Autodesk Inventor part; units mm, degrees
ref_plane "YZ Plane" through (0, 0, 0) normal (1, 0, 0) x (0, 1, 0)
ref_plane "XZ Plane" through (0, 0, 0) normal (0, 1, 0) x (-1, 0, 0)
ref_plane "XY Plane" through (0, 0, 0) normal (0, 0, 1) x (1, 0, 0)
sketch "Sketch1" plane through (0, 0, 0) normal (0, 1, 0) x (-1, 0, 0)
  line L0 (35.2615, 31.9433) -> (-167.9385, 31.9433)
  line L1 (-167.9385, 31.9433) -> (-167.9385, -69.6567)
  line L2 (-167.9385, -69.6567) -> (35.2615, -69.6567)
  line L3 (35.2615, -69.6567) -> (35.2615, 31.9433)
  line L4 (-167.9385, 31.9433) -> (-218.7385, 31.9433)
  line L5 (-218.7385, 31.9433) -> (-218.7385, 6.5433)
  line L6 (-218.7385, 6.5433) -> (-167.9385, 6.5433)
  line L7 (-167.9385, 6.5433) -> (-167.9385, 31.9433)
  line L8 (-167.9385, -69.6567) -> (-218.7385, -69.6567)
  line L9 (-218.7385, -69.6567) -> (-218.7385, -44.2567)
  line L10 (-218.7385, -44.2567) -> (-167.9385, -44.2567)
  line L11 (-167.9385, -44.2567) -> (-167.9385, -69.6567)
  point P0 (0, 0)
  point P1 (-167.9385, 6.5433)
  dimension "d0" = 101.6
  dimension "d1" = 203.2
  dimension "d2" = 50.8
  dimension "d3" = 50.8
extrude "Extrusion1" add sketch "Sketch1" along normal blind 38.1 contours L1 L6 L5 L4 | L8 L9 L10 L1
extrude "Extrusion2" add sketch "Sketch1" along normal blind 25.4 contours L3 L2 L1 L0
sketch "Sketch2" plane through (167.9385, 38.1, 31.9433) normal (0, 0, 1) x (1, 0, 0)
  line L0 (50.8, -38.1) -> (50.8, 0) construction
  line L1 (0, 0) -> (50.8, 0) construction
  line L2 (50.8, -19.05) -> (31.75, -19.05) construction
  line L3 (31.75, -19.05) -> (31.75, 0) construction
  line L4 (31.75, 0) -> (50.8, 0) construction
  line L5 (50.8, 0) -> (50.8, -19.05) construction
  circle A0 centre (31.75, -19.05) radius 12.7
  point P0 (-167.9385, -38.1)
  dimension "d8" = 25.4
extrude "Extrusion3" add sketch "Sketch2" against normal through all
fillet "Fillet1" radius 12.7 6 edges at (167.9385, 38.1, 19.2433) (167.9385, 38.1, -56.9567) (218.7385, 38.1, 19.2433) (218.7385, 38.1, -56.9567) (218.7385, 0, 19.2433) (218.7385, 0, -56.9567)
fillet "Fillet2" radius 6.35 2 edges at (-35.2615, 25.4, -18.8567) (-35.2615, 0, -18.8567)
properties part number "Pedals"
Source: CAD feature listing. Evaluate the final solid. Frame: model axes, mm. A direction names the side the tool comes from. Give positions to 0.01 mm unless a question says otherwise; leave off trailing zeros. Loops run counter-clockwise (first coordinate to the right, second up) from the corner with the lowest first, then second, coordinate; pieces in that order, holes last. Notation, with made-up numbers: (31, 74.25) -> (83, 74.25) arc R16 cw to (83, 97.25) -> close; hole circle Ø1 at (-2.75, 58.25). An arc over 180 degrees is marked (long way). Put each result on its own line as item: value. Start each with the question number.
1) Contact query for flat-ended pins moving along their axis: P1, Ø1.5, axis at y = 33, z = -48.5, coming from the +X side; P2, Ø2, axis at x = 176.5, z = 5.5, coming from the +Y side; P3, Ø10, axis at x = -0.5, z = -46, coming from the +Y side; P4, Ø2, axis at y = 33.5, z = -56, coming from the -X side. Output: stop coordinate, or through.
2) Cut plane B-B (y = 23). Return loops of the section in (x, z), then the cut area to 3 significant figures.
3) Cut plane D-D (x = 18). Return loops of the section in (y, z).
4) Reachability of faces 1 (the face through (188, 10, 6.543)), 2 (the face through (167.938, 13, -19)), 3 (the face through (71, 25.4, -18)) from +Z, -Z, +X, -X, +Y, -Y: full face, straight path, thin tool, end or side. Return the list, or none.
5) Material intervals for probe 1 along Z at (x, y) = (194, 35); probe 2 along X at (y, z) = (18, -29); probe 3 along Y at (x, z) = (103, -43.5), sorted ascending.
6) Draft query along Z for faces 4 (the face through (90, 15, 31.943)), 5 (the face through (90, 0, -18)), 6 (the face through (188, 10, -44.257)). Return one class per face: released by +Z, released by -Z, zero draft, split by the parting line, or undercut.
7) Cut plane A-A (z = -13). Return loops of the section in (x, y), then the cut area to 3 significant figures.
Results are:
1. P1: stops at x = 216.73
1. P2: passes through
1. P3: stops at y = 25.4
1. P4: stops at x = 170.11
2. outline: (-33.88, -69.66) -> (218.74, -69.66) -> (218.74, -44.26) -> (211.76, -44.26) -> (211.76, 6.54) -> (218.74, 6.54) -> (218.74, 31.94) -> (-33.88, 31.94) -> close; hole (167.94, -44.26) -> (187.62, -44.26) -> (187.62, 6.54) -> (167.94, 6.54) -> close
2. area: 24,300 mm2
3. outline: (0, -69.66) -> (25.4, -69.66) -> (25.4, 31.94) -> (0, 31.94) -> close
4. face 1: none
4. face 2: +Y, -Y
4. face 3: +Z, -Z, -X, +Y
5. probe 1: z = -69.66 to -44.26, 6.54 to 31.94
5. probe 2: x = -35.26 to 167.94, 187.03 to 212.35
5. probe 3: y = 0 to 25.4
6. face 4: released by +Z
6. face 5: zero draft
6. face 6: undercut
7. outline: (-35.26, 6.35) arc R6.35 ccw to (-28.91, 0) -> (167.94, 0) -> (167.94, 25.4) -> (-28.91, 25.4) arc R6.35 ccw to (-35.26, 19.05) -> close; circle Ø25.4 at (199.69, 19.05)
7. area: 5,650 mm2
